Verification items for this drawing (mm, ordinates from the low corner). A direction names the side the tool comes from. Round coordinates to 2 decimals unless told otherwise and drop trailing zeros. Loops run counter-clockwise (first coordinate to the right, second up) from the corner with the lowest first, then second, coordinate; pieces in that order, holes last. Notation, with made-up numbers: M -1.5,5.25 L 21.5,5.25 A13 cw 21.5,9.25 Z; hole C 35,-6.75 d9. An arc over 180 degrees is marked long. Answer as CSV lines item,"result".
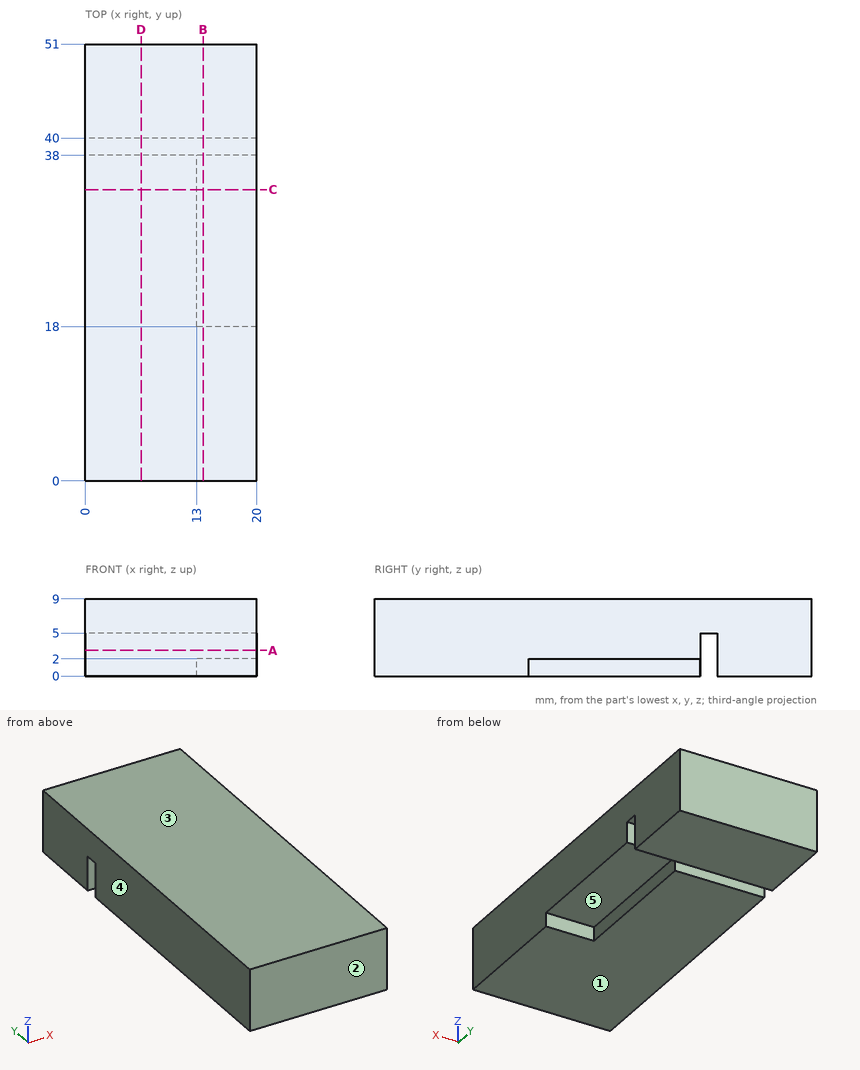
1) Draft check along Z on the marked faces 1, 2 and 3. Enter one of: +Z half, -Z half, draft (parallel to the pull), parting line (faces both ways), or undercut.
Here are the results:
face 1,"-Z half"
face 2,"draft"
face 3,"+Z half"
2) Section check D-D (x = 6.5). Record the cut outline in (y, z), plus the area to 3 significant figures.
Here are the results:
outline,"M 0,0 L 38,0 L 38,5 L 40,5 L 40,0 L 51,0 L 51,9 L 0,9 Z"
area,"449 mm^2"
3) Section check C-C (y = 34). Record the cut outline in (x, z), plus the area to 3 significant figures.
Here are the results:
outline,"M 0,0 L 13,0 L 13,2 L 20,2 L 20,9 L 0,9 Z"
area,"166 mm^2"
4) Section check A-A (z = 3). Record the cut outline in (x, y).
Here are the results:
outline,"M 0,0 L 20,0 L 20,38 L 0,38 Z; M 0,40 L 20,40 L 20,51 L 0,51 Z"
5) Section check B-B (x = 13.75). Record the cut outline in (y, z).
Here are the results:
outline,"M 0,0 L 18,0 L 18,2 L 38,2 L 38,5 L 40,5 L 40,0 L 51,0 L 51,9 L 0,9 Z"
6) Go/stop test with flat-tipped pins: pin 1 (2 mm diameter, centred on x = 17.5, y = 28, fed in from -Z); pin 2 (0.6 mm diameter, centred on y = 26.5, z = 0.5, fed in from +X); pin 3 (0.6 mm diameter, centred on x = 5, y = 39.5, fed in from -Z). Record where each tip stops, or that it passes through.
Here are the results:
pin 1,"stops at z = 2"
pin 2,"stops at x = 13"
pin 3,"stops at z = 5"
7) Material ranges on probe 1 along Y at (x, z) = (2, 2.75); probe 2 along Y at (x, z) = (15.75, 1); probe 3 along Z at (x, y) = (18.5, 22.5), recorded low to high.
Here are the results:
probe 1,"y = 0 to 38, 40 to 51"
probe 2,"y = 0 to 18, 40 to 51"
probe 3,"z = 2 to 9"
8) Set-up check for the marked faces 4 and 5: record each of +Z, -Z, +X, -X, +Y, -Y from which the full face is reachable in a straight line by a thin tool's end or side.
Here are the results:
face 4,"+Z, -Z, -X, +Y, -Y"
face 5,"-Z, +X"
